Geometry: final body of the model. Coordinates: model frame, mm. Face numbers are marked on the shaded views. A direction names the side the tool comes from. Round coordinates to 2 decimals unless told otherwise and drop trailing zeros. Write each loop counter-clockwise with the first axis right and the second up, starting at its lowest first coordinate (ties: lowest second). Pieces come first, ordered by that corner, then holes.
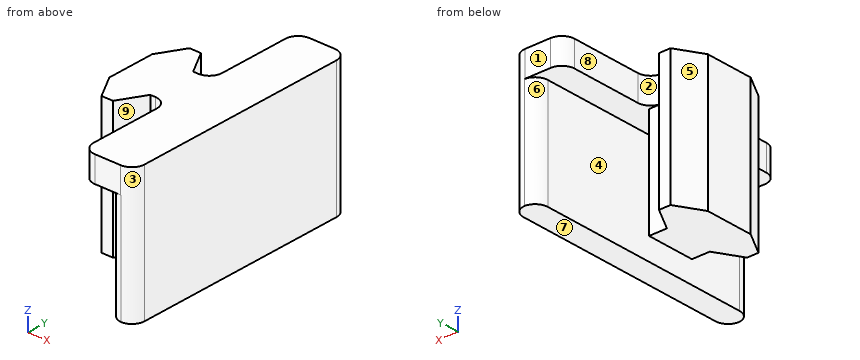
from build123d import *

# Parameters (mm, degrees)
SALIENTE_EXTRUIR1_DEPTH = 21
CROQUIS3_W              = 4.2
CROQUIS3_H              = 38
CORTAR_EXTRUIR1_DEPTH   = 17
REDONDEO1_R             = 2


with BuildPart() as part:
    # Croquis1 → Saliente-Extruir1 (new body)
    with BuildSketch(Plane(origin=(0, 0, 0), x_dir=(0, 1, 0), z_dir=(0, 0, 1))):
        Polygon((-3.8, 9.209401077), (3.8, 9.209401077), (7.8, 6.9), (7.8, 5.1), (3.8, 2.790598923), (3.8, 0), (19, 0), (19, -8), (-19, -8), (-19, 0), (-3.8, 0), (-3.8, 2.790598923), (-7.8, 5.1), (-7.8, 6.9), align=None)
    extrude(amount=SALIENTE_EXTRUIR1_DEPTH)

    # Croquis3 → Cortar-Extruir1 (cut)
    with BuildSketch(Plane(origin=(0, 0, 0), x_dir=(1, 0, 0), z_dir=(0, 0, -1))):
        with Locations((2.1, 0)):
            Rectangle(CROQUIS3_W, CROQUIS3_H)
    extrude(amount=-CORTAR_EXTRUIR1_DEPTH, mode=Mode.SUBTRACT)

    # Redondeo1
    # the kernel refuses this fillet: 2 mm, written as the material it adds along each edge
    with BuildSketch(Plane(origin=(0, -3.8, 17), x_dir=(-1, 0, 0), z_dir=(0, 0, 1))) as redondeo1_piece_1:
        with BuildLine():
            CenterArc((REDONDEO1_R, REDONDEO1_R), REDONDEO1_R, 180, 90)
            Line((0, REDONDEO1_R), (0, 0))
            Line((0, 0), (REDONDEO1_R, 0))
        make_face()
    extrude(amount=4)
    with BuildSketch(Plane(origin=(0, 3.8, 17), x_dir=(-1, 0, 0), z_dir=(0, 0, 1))) as redondeo1_piece_2:
        with BuildLine():
            CenterArc((REDONDEO1_R, -REDONDEO1_R), REDONDEO1_R, 90, 90)
            Line((0, -REDONDEO1_R), (0, 0))
            Line((0, 0), (REDONDEO1_R, 0))
        make_face()
    extrude(amount=4)
    # the kernel refuses this fillet: 2 mm, written as the material it takes off along each edge
    with BuildSketch(Plane(origin=(8, 19, -5), x_dir=(-1, 0, 0), z_dir=(0, 0, 1)), Plane(origin=(8, -19, -5), x_dir=(0, 1, 0), z_dir=(0, 0, 1))) as redondeo1_2_piece_1:
        with BuildLine():
            CenterArc((REDONDEO1_R, REDONDEO1_R), REDONDEO1_R, 180, 90)
            Line((0, REDONDEO1_R), (0, 0))
            Line((0, 0), (REDONDEO1_R, 0))
        make_face()
    extrude(amount=31, mode=Mode.SUBTRACT)
    with BuildSketch(Plane(origin=(4.2, -19, -5), x_dir=(1, 0, 0), z_dir=(0, 0, 1))) as redondeo1_2_piece_2:
        with BuildLine():
            CenterArc((REDONDEO1_R, REDONDEO1_R), REDONDEO1_R, 180, 90)
            Line((0, REDONDEO1_R), (0, 0))
            Line((0, 0), (REDONDEO1_R, 0))
        make_face()
    extrude(amount=22, mode=Mode.SUBTRACT)
    with BuildSketch(Plane(origin=(0, -19, 12), x_dir=(1, 0, 0), z_dir=(0, 0, 1)), Plane(origin=(0, 19, 12), x_dir=(0, -1, 0), z_dir=(0, 0, 1))) as redondeo1_2_piece_3:
        with BuildLine():
            CenterArc((REDONDEO1_R, REDONDEO1_R), REDONDEO1_R, 180, 90)
            Line((0, REDONDEO1_R), (0, 0))
            Line((0, 0), (REDONDEO1_R, 0))
        make_face()
    extrude(amount=14, mode=Mode.SUBTRACT)
    with BuildSketch(Plane(origin=(4.2, 19, -5), x_dir=(1, 0, 0), z_dir=(0, 0, 1))) as redondeo1_2_piece_4:
        with BuildLine():
            CenterArc((REDONDEO1_R, -REDONDEO1_R), REDONDEO1_R, 90, 90)
            Line((0, -REDONDEO1_R), (0, 0))
            Line((0, 0), (REDONDEO1_R, 0))
        make_face()
    extrude(amount=22, mode=Mode.SUBTRACT)


solid = part.part
1) Section D-D on y = -15.5. Output: boundary loops of the cut face in (x, z), plus the area to 3 significant figures.
2) Section C-C on x = 5. Output: boundary loops of the cut face in (y, z).
3) Section B-B on y = 5. Output: boundary loops of the cut face in (x, z).
4) Draft query along X for the marked faces 1, 2, 3 and 4. Return one class per face: pulls with the +X half, pulls with the -X half, needs draft (parallel to the pull), parting line crosses it, or undercut.
5) Line query: probe 1 along X at (y, z) = (-1, 6.25); probe 2 along X at (y, z) = (10.5, 9.5); probe 3 along Z at (x, y) = (4, 14). Output: solid intervals per line, ascending.
6) First-contact query: P1, Ø2, axis at y = -11, z = 19.5, coming from the -X side; P2, Ø2, axis at x = -6.5, z = 11, coming from the -Y side; P3, Ø2, axis at x = 2, y = 7.5, coming from the -Z side. Flat tips, straight axial feed; report the tip coordinate or a pass-through.
7) Reachability of the marked faces 5, 6, 7, 8 and 9 from +Z, -Z, +X, -X, +Y, -Y: full face, straight path, thin tool, end or side. Return the list, or none.
8) Section A-A on z = 2.5. Output: boundary loops of the cut face in (x, y).
Filled in:
1. outline: (0, 17) - (4.2, 17) - (4.2, 0) - (8, 0) - (8, 21) - (0, 21) - close
1. area: 96.6 mm2
2. outline: (-19, 17) - (-18.6, 17) - (-18.6, 0) - (18.6, 0) - (18.6, 17) - (19, 17) - (19, 21) - (-19, 21) - close
3. outline: (-8.52, 0) - (-3.48, 0) - (-3.48, 21) - (-8.52, 21) - close; (-0.17, 17) - (4.2, 17) - (4.2, 0) - (8, 0) - (8, 21) - (-0.17, 21) - close
4. face 1: needs draft
4. face 2: undercut
4. face 3: pulls with the +X half
4. face 4: undercut
5. probe 1: x = -9.21 to 0, 4.2 to 8
5. probe 2: x = 4.2 to 8
5. probe 3: z = 17 to 21
6. P1: stops at x = 0
6. P2: stops at y = -7.8
6. P3: stops at z = 17
7. face 5: +Z, -Z, -X, +Y
7. face 6: -Z, -X, +Y
7. face 7: -Z, +X, -X, +Y, -Y
7. face 8: +Z, -Z, +Y
7. face 9: +Z, -Z, -Y
8. outline: (-9.21, -3.8) - (-6.9, -7.8) - (-5.1, -7.8) - (-2.79, -3.8) - (0, -3.8) - (0, 3.8) - (-2.79, 3.8) - (-5.1, 7.8) - (-6.9, 7.8) - (-9.21, 3.8) - close; (4.2, -17) arc R2 ccw to (6.1, -19) arc R2 ccw to (8, -17) - (8, 17) arc R2 ccw to (6.1, 19) arc R2 ccw to (4.2, 17) - close
